from build123d import *

# Parameters (mm, degrees)
SKETCH_5_R          = 11.5
SKETCH_5_R_2        = 1.35
EXTRUDE_3_DEPTH     = 3
SKETCH_8_W          = 33
SKETCH_8_H          = 3
EXTRUDE_4_DEPTH     = 30
SKETCH_10_R         = 1.6
CUT_EXTRUDE_4_DEPTH = 5
FILLET_1_R          = 2
FILLET_2_R          = 5
CHAMFER_1_SIZE      = 2


with BuildPart() as part:
    # 草图5 → 凸台-拉伸3 (new body)
    with BuildSketch(Plane(origin=(0, 0, 0), x_dir=(1, 0, 0), z_dir=(0, 1, 0))):
        Polygon((16.5, 23.5), (16.5, -14.5), (14.5, -16.5), (-14.5, -16.5), (-16.5, -14.5), (-16.5, 23.5), align=None)
        with Locations(Location((0, 0, 0), (0, 0, 270))):
            Circle(SKETCH_5_R, mode=Mode.SUBTRACT)
        with Locations(Location((-11.5, -11.5, 0), (0, 0, 270))):
            Circle(SKETCH_5_R_2, mode=Mode.SUBTRACT)
        with Locations(Location((-11.5, 11.5, 0), (0, 0, 270))):
            Circle(SKETCH_5_R_2, mode=Mode.SUBTRACT)
        with Locations(Location((11.5, 11.5, 0), (0, 0, 270))):
            Circle(SKETCH_5_R_2, mode=Mode.SUBTRACT)
        with Locations(Location((11.5, -11.5, 0), (0, 0, 270))):
            Circle(SKETCH_5_R_2, mode=Mode.SUBTRACT)
    extrude(amount=EXTRUDE_3_DEPTH)

    # 草图8 → 凸台-拉伸4 (add)
    with BuildSketch(Plane(origin=(0, 3, 0), x_dir=(1, 0, 0), z_dir=(0, 1, 0))):
        with Locations((0, 22)):
            Rectangle(SKETCH_8_W, SKETCH_8_H)
    extrude(amount=EXTRUDE_4_DEPTH)

    # 草图10 → 切除-拉伸4 (cut)
    with BuildSketch(Plane.XY.offset(-20.5)):
        with Locations((-7.5, 23)):
            Circle(SKETCH_10_R)
        with Locations((7.5, 23)):
            Circle(SKETCH_10_R)
        with Locations((7.5, 13)):
            Circle(SKETCH_10_R)
        with Locations((-7.5, 13)):
            Circle(SKETCH_10_R)
        with Locations((-10, 18)):
            Circle(SKETCH_10_R)
        with Locations((10, 18)):
            Circle(SKETCH_10_R)
    extrude(amount=-CUT_EXTRUDE_4_DEPTH, mode=Mode.SUBTRACT)

    # 圆角1
    fillet_1_edges = [part.edges().sort_by_distance(p)[0] for p in [
        (0, 3, -20.5),
    ]]
    fillet(fillet_1_edges, radius=FILLET_1_R)

    # 圆角2
    fillet_2_edges = [part.edges().sort_by_distance(p)[0] for p in [
        (0, 0, -23.5),
    ]]
    fillet(fillet_2_edges, radius=FILLET_2_R)

    # 倒角1
    chamfer_1_edges = [part.edges().sort_by_distance(p)[0] for p in [
        (-16.5, 33, -22),
        (16.5, 33, -22),
    ]]
    chamfer(chamfer_1_edges, length=CHAMFER_1_SIZE)


solid = part.part
CAD build for the part. Positions are in the model's coordinates, mm. A direction names the side the tool comes from. Round coordinates to 2 decimals unless told otherwise and drop trailing zeros. Write each loop counter-clockwise with the first axis right and the second up, starting at its lowest first coordinate (ties: lowest second). Pieces come first, ordered by that corner, then holes.
(1) Slice it at B-B, the plane z = 0. Write the cut outline in (x, y), and give its area (3 significant figures).
(2) Slice it at A-A, the plane y = 13. Write the cut outline in (x, z), and give its area (3 significant figures).
(3) Slice it at C-C, the plane x = 0. Write the cut outline in (y, z), and give its area (3 significant figures).
(4) Mould opens along Z. For faces 1 (the face through (16, 1, 15)), 2 (the face through (-15.5, 32, -22)), 3 (the face through (-10.161, 1.479, 11.324)) say: pulls with the +Z half, pulls with the -Z half, needs draft (parallel to the pull), parting line crosses it, or undercut.
(5) 3-axis set-ups, long thin cutter, end or side, ignore diameter. For faces 4 (the face through (8, 3, -9)), 5 (the face through (-10.161, 1.479, -11.676)): which of +Z, -Z, +X, -X, +Y, -Y reach the whole face in a straight line?
(6) Drop flat-ended pins along their axis: P1, Ø8.5, axis at x = 2.5, y = 16, coming from the +Z side; P2, Ø1, axis at x = 10.5, z = -12.5, coming from the +Y side. Give the stop position or say it passes through.
(7) Probe line 1 along Y through (x, z) = (7.5, -21.3); line 2 along Y through (x, z) = (3, -15.5); line 3 along Z through (x, y) = (-2.5, 19). List the from-to ranges inside material, lowest first.
(8) Slice it at D-D, the plane x = -7.5. Write the cut outline in (y, z), and give its area (3 significant figures).
From the geometry:
1. outline: (-16.5, 0) - (-11.5, 0) - (-11.5, 3) - (-16.5, 3) - close; (11.5, 0) - (16.5, 0) - (16.5, 3) - (11.5, 3) - close
1. area: 30.0 mm2
2. outline: (-16.5, -23.5) - (-9.1, -23.5) - (-9.1, -20.5) - (-16.5, -20.5) - close; (-5.9, -23.5) - (5.9, -23.5) - (5.9, -20.5) - (-5.9, -20.5) - close; (9.1, -23.5) - (16.5, -23.5) - (16.5, -20.5) - (9.1, -20.5) - close
2. area: 79.8 mm2
3. outline: (0, -18.5) arc R5 ccw to (5, -23.5) - (33, -23.5) - (33, -20.5) - (5, -20.5) arc R2 cw to (3, -18.5) - (3, -11.5) - (0, -11.5) - close; (0, 11.5) - (3, 11.5) - (3, 16.5) - (0, 16.5) - close
3. area: 136 mm2
4. face 1: pulls with the +Z half
4. face 2: needs draft
4. face 3: undercut
5. face 4: +Z, +X, -X, +Y
5. face 5: +Y, -Y
6. P1: stops at z = -20.5
6. P2: stops at y = 3
7. line 1: y = 0.86 to 11.4, 14.6 to 21.4, 24.6 to 33
7. line 2: y = 0 to 3
7. line 3: z = -23.5 to -20.5
8. outline: (0, -18.5) arc R5 ccw to (5, -23.5) - (11.4, -23.5) - (11.4, -20.5) - (5, -20.5) arc R2 cw to (3, -18.5) - (3, -8.72) - (0, -8.72) - close; (0, 8.72) - (3, 8.72) - (3, 16.5) - (0, 16.5) - close; (14.6, -23.5) - (21.4, -23.5) - (21.4, -20.5) - (14.6, -20.5) - close; (24.6, -23.5) - (33, -23.5) - (33, -20.5) - (24.6, -20.5) - close
8. area: 134 mm2
